Autodesk Inventor part; units mm, degrees
ref_plane "YZ Plane" through (0, 0, 0) normal (1, 0, 0) x (0, 1, 0)
ref_plane "XZ Plane" through (0, 0, 0) normal (0, 1, 0) x (-1, 0, 0)
ref_plane "XY Plane" through (0, 0, 0) normal (0, 0, 1) x (1, 0, 0)
sketch "Sketch1" plane through (0, 0, 0) normal (0, 0, 1) x (1, 0, 0)
  line L0 (0, 0) -> (-375, 0)
  line L1 (-375, 0) -> (-375, -600)
  line L2 (-375, -600) -> (0, -600)
  line L3 (0, -600) -> (0, 0)
  line L4 (-405, 30) -> (30, 30)
  line L5 (30, 30) -> (30, -630)
  line L6 (30, -630) -> (-405, -630)
  line L7 (-405, -630) -> (-405, 30)
  line L8 (-405, -630) -> (-375, -630)
  line L9 (-375, -630) -> (-375, -1270)
  line L10 (-375, -1270) -> (-405, -1270)
  line L11 (-405, -1270) -> (-405, -630)
  line L12 (30, -630) -> (0, -630)
  line L13 (0, -630) -> (0, -1270)
  line L14 (0, -1270) -> (30, -1270)
  line L15 (30, -1270) -> (30, -630)
  line L16 (-375, -1270) -> (0, -1270)
  line L17 (0, -1270) -> (0, -1240)
  line L18 (0, -1240) -> (-375, -1240)
  line L19 (-375, -1240) -> (-375, -1270)
  dimension "d0" = 375
  dimension "d1" = 600
  dimension "d2" = 30
  dimension "d3" = 30
  dimension "d4" = 30
  dimension "d5" = 30
  dimension "d38" = 30
  dimension "d39" = 640
  dimension "d40" = 30
  dimension "d41" = 640
  dimension "d42" = 30
extrude "Extrusion1" add sketch "Sketch1" along normal blind 30 contours L4 L5 L6 L7
sketch "Sketch2" plane through (0, 0, 0) normal (0, 0, -1) x (-1, 0, 0)
  line L0 (375, -600) -> (375, 0)
  line L1 (375, -450) -> (0, -450)
  line L2 (0, -450) -> (0, -410)
  line L3 (0, -410) -> (375, -410)
  line L4 (375, -410) -> (375, -450)
  line L5 (0, -600) -> (375, -600)
  line L6 (202.5, -600) -> (202.5, -450)
  line L7 (172.5, -600) -> (172.5, -450)
  point P0 (0, 0)
  dimension "d8" = 375
  dimension "d9" = 40
  dimension "d10" = 150
extrude "Extrusion2" add sketch "Sketch2" against normal blind 30 contours L1 L2 L3 L0 | L5 L7 L1 L6
sketch "Sketch3" plane through (0, 0, 30) normal (0, 0, 1) x (1, 0, 0)
  line L0 (12.5, -490) -> (17.5, -490)
  line L1 (17.5, -490) -> (17.5, -200)
  line L2 (17.5, -200) -> (12.5, -200)
  line L3 (12.5, -200) -> (12.5, -490)
  line L4 (0, -410) -> (-375, -410)
  line L5 (-392.5, -490) -> (-387.5, -490)
  line L6 (-387.5, -490) -> (-387.5, -200)
  line L7 (-387.5, -200) -> (-392.5, -200)
  line L8 (-392.5, -200) -> (-392.5, -490)
  line L9 (0, -600) -> (-172.5, -600)
  point P0 (0, 0)
  dimension "d13" = 5
  dimension "d14" = 290
  dimension "d18" = 405
  dimension "d37" = 110
extrude "Extrusion3" [suppressed]
sketch "Sketch4" plane through (30, -630, 0) normal (1, 0, 0) x (0, 0, -1)
  line L0 (-30, 0) -> (-30, 660)
  line L1 (-30, 660) -> (-657.8518, 828.2324)
  line L2 (-30, 660) -> (620, 660) construction
  line L3 (-657.8518, 828.2324) -> (-665.6164, 799.2546)
  line L4 (-665.6164, 799.2546) -> (-30, 628.9417)
  point P0 (0, 630)
  dimension "d25" = 650
  dimension "d26" = 165
  dimension "d27" = 30
  dimension "d28" = 270
extrude "Extrusion4" [suppressed]
pattern_linear "Rectangular Pattern1" [suppressed]
sketch "Sketch5" plane through (-375, 0, 30) normal (1, 0, 0) x (0, 0, -1)
  line L0 (-635.6164, 169.2546) -> (-627.8518, 198.2324)
  line L1 (0, -1.0583) -> (-635.6164, 169.2546)
  line L2 (-627.8518, 198.2324) -> (-635.6164, 169.2546)
  line L3 (-635.6164, 169.2546) -> (-606.6386, 161.49)
  line L4 (-606.6386, 161.49) -> (-598.874, 190.4678)
  line L5 (-627.8518, 198.2324) -> (0, 30)
  line L6 (-627.8518, 198.2324) -> (-598.874, 190.4678)
  point P0 (30, 0)
  dimension "d34" = 30
extrude "Extrusion5" [suppressed]
sketch "Sketch6" plane through (0, 0, 0) normal (0, 0, -1) x (-1, 0, 0)
  line L0 (0, -630) -> (0, -1270)
  line L1 (0, -1270) -> (-30, -1270)
  line L2 (-30, -1270) -> (-30, -630)
  line L3 (375, -630) -> (375, -1270)
  line L4 (375, -1270) -> (405, -1270)
  line L5 (405, -1270) -> (405, -630)
  line L6 (0, -1270) -> (375, -1270)
  line L7 (375, -1270) -> (375, -1240)
  line L8 (375, -1240) -> (0, -1240)
  line L9 (0, -1240) -> (0, -1270)
  line L10 (405, 30) -> (405, -630)
  line L11 (-30, -630) -> (-30, 30)
  line L12 (405, -630) -> (375, -630)
  line L13 (405, -630) -> (-30, -630)
  line L14 (0, -630) -> (-30, -630)
  point P0 (0, 0)
  point P1 (405, -1.0583)
  point P2 (-30, -1.0583)
  dimension "d43" = 30
  dimension "d44" = 640
  dimension "d45" = 30
  dimension "d46" = 640
  dimension "d47" = 30
  dimension "d48" = 0
  dimension "d49" = 0
extrude "Extrusion6" add sketch "Sketch6" against normal blind 30 contours L0 L1 L2 L13 | L8 L3 L6 L0 | L12 L5 L4 L3
sketch "Sketch7" plane through (0, 0, 0) normal (0, 0, -1) x (-1, 0, 0)
  circle A0 centre (187.5, -430) radius 40
  point P0 (0, 0)
  dimension "d52" = 80
sketch "Sketch8" plane through (30, -1270, 0) normal (1, 0, 0) x (0, 0, -1)
  line L0 (0, 0) -> (-30, 0)
  line L1 (-30, 0) -> (-311.9078, 102.606)
  line L2 (-30, 0) -> (270, 0) construction
  line L3 (-311.9078, 102.606) -> (-301.6472, 130.7968)
  line L4 (-301.6472, 130.7968) -> (-30, 31.9253)
  line L5 (-30, 640) -> (-30, 30)
  line L6 (-30, 31.9253) -> (-30, 0)
  point P0 (0, 1270)
  dimension "d55" = 300
  dimension "d56" = 160
  dimension "d57" = 30
  dimension "d58" = 90
sketch "Sketch9" plane through (0, -1240, 0) normal (-1, 0, 0) x (0, 0, 1)
  line L0 (311.9078, 72.606) -> (301.6472, 100.7968)
  line L1 (311.9078, 72.606) -> (301.6472, 100.7968)
  line L2 (301.6472, 100.7968) -> (273.4564, 90.5362)
  line L3 (30, 1.9253) -> (301.6472, 100.7968)
  line L4 (273.4564, 90.5362) -> (283.717, 62.3454)
  line L5 (30, -30) -> (311.9078, 72.606)
  line L6 (283.717, 62.3454) -> (311.9078, 72.606)
  point P0 (0, 1240)
  dimension "d64" = 30
sketch "Sketch10" plane through (0, 0, 30) normal (0, 0, 1) x (1, 0, 0)
  line L0 (-405, -1238.0747) -> (-375, -1238.0747)
  line L1 (-405, -1238.0747) -> (30, -1238.0747)
  line L2 (30, -1238.0747) -> (30, -598.0747)
  line L3 (30, -598.0747) -> (-405, -598.0747)
  line L4 (-405, -598.0747) -> (-405, -1238.0747)
  point P0 (0, 0)
  dimension "d67" = 435
  dimension "d68" = 640
sketch "Sketch11" plane through (0, 0, 32) normal (0, 0, 1) x (1, 0, 0)
  line L0 (30, -648.0747) -> (0, -648.0747)
  line L1 (0, -648.0747) -> (0, -678.0747)
  line L2 (0, -678.0747) -> (30, -678.0747)
  line L3 (30, -678.0747) -> (30, -648.0747)
  line L4 (30, -598.0747) -> (-405, -598.0747)
  point P0 (0, 0)
  dimension "d71" = 30
  dimension "d72" = 30
  dimension "d73" = 50
sketch "Sketch12" plane through (0, 0, 382) normal (0, 0, 1) x (1, 0, 0)
  line L0 (-405, -868.0747) -> (-405, -898.0747)
  line L1 (-405, -898.0747) -> (-375, -898.0747)
  line L2 (-375, -898.0747) -> (-375, -868.0747)
  line L3 (-375, -868.0747) -> (-405, -868.0747)
  line L4 (-405, -648.0747) -> (-405, -678.0747)
  line L5 (-405, -678.0747) -> (-375, -678.0747)
  line L6 (-375, -678.0747) -> (-375, -648.0747)
  line L7 (-375, -648.0747) -> (-405, -648.0747)
  line L8 (0, -648.0747) -> (0, -678.0747)
  line L9 (0, -678.0747) -> (30, -678.0747)
  line L10 (30, -678.0747) -> (30, -648.0747)
  line L11 (30, -648.0747) -> (0, -648.0747)
  line L12 (0, -868.0747) -> (0, -898.0747)
  line L13 (0, -898.0747) -> (30, -898.0747)
  line L14 (30, -898.0747) -> (30, -868.0747)
  line L15 (30, -868.0747) -> (0, -868.0747)
  line L16 (-405, -898.0747) -> (-375, -898.0747)
  line L17 (-405, -898.0747) -> (30, -898.0747)
  line L18 (30, -898.0747) -> (30, -648.0747)
  line L19 (30, -648.0747) -> (-405, -648.0747)
  line L20 (-405, -648.0747) -> (-405, -898.0747)
  point P0 (0, 0)
  point P1 (0, -898.0747)
  point P2 (30, -868.0747)
  point P3 (30, -678.0747)
  point P4 (0, -648.0747)
sketch "Sketch13" plane through (-405, -1270, 0) normal (-1, 0, 0) x (0, 0, 1)
  line L0 (232, 591.9253) -> (202, 591.9253)
  line L1 (202, 591.9253) -> (202, 741.9253)
  line L2 (202, 741.9253) -> (232, 741.9253)
  line L3 (232, 741.9253) -> (232, 591.9253)
  line L4 (32, 591.9253) -> (379, 591.9253)
  line L5 (382, 621.9253) -> (382, 371.9253)
  point P0 (0, 1270)
  dimension "d84" = 30
  dimension "d85" = 150
  dimension "d86" = 0
  dimension "d87" = 150
sketch "Sketch14" plane through (-435, -1270, 0) normal (-1, 0, 0) x (0, 0, 1)
  line L0 (232, 741.9253) -> (202, 741.9253)
  line L1 (232, 741.9253) -> (202, 741.9253)
  line L2 (202, 741.9253) -> (202, 711.9253)
  line L3 (202, 711.9253) -> (232, 711.9253)
  line L4 (232, 711.9253) -> (232, 741.9253)
  point P0 (0, 1270)
  point P1 (202, 741.9253)
  dimension "d90" = 30
  dimension "d91" = 30
sketch "Sketch15" plane through (30, -1270, 0) normal (1, 0, 0) x (0, 0, -1)
  line L0 (-657.8518, 1468.2324) -> (-665.6164, 1439.2546) construction
  circle A0 centre (-661.7341, 1453.7435) radius 7.5 construction
  circle A1 centre (-654.5905, 1451.4588) radius 4
  point P0 (0, 1270)
  dimension "d96" = 15
  dimension "d97" = 8
properties part number "rama pod fotel v2 bez mocowań kierownicy"
Can you work these out from the model? Positions are in its coordinate system, mm. A direction names the side the tool comes from. Coordinates: 2 decimals unless noted, no trailing zeros. Order: outer loops, then holes, each group sorted by start corner. A loop starts at its lowest first (then second) coordinate and runs counter-clockwise, first axis right, second up.
1. If we section it at A-A (x = -77): Please give me the cut outline in (y, z), then the cut area to 3 significant figures.
2. For faces 5 (the face through (0, -526, 15)), 6 (the face through (-189, -617, 30)), which set-ups out of +Z, -Z, +X, -X, +Y, -Y let a thin tool reach every point of the face, with its end or its side?
3. If we section it at B-B (y = -1051): Please give me the cut outline in (x, z).
4. I need wall thicknesses on line 1 (Y direction, x = -225, z = 11); line 2 (X direction, y = -521.5, z = 19.5); line 3 (Y direction, x = -184.5, z = 10.75). Which ranges of each line are inside material? Lowest first, please.
5. Thinking about a two-plate mould opening in X: for faces 1 (the face through (-405, -629, 15)), 2 (the face through (-290, -600, 15)), 3 (the face through (-191, -1270, 15)), 4 (the face through (-185, -630, 15)), which applies, +X half, -X half, draft (parallel to the pull), parting line (faces both ways), or undercut?
6. If we section it at C-C (z = 5): Please give me the cut outline in (x, y).
Entries:
1. outline: (-1270, 0) - (-1240, 0) - (-1240, 30) - (-1270, 30) - close; (-630, 0) - (-600, 0) - (-600, 30) - (-630, 30) - close; (-450, 0) - (-410, 0) - (-410, 30) - (-450, 30) - close; (0, 0) - (30, 0) - (30, 30) - (0, 30) - close
1. area: 3,900 mm2
2. face 5: +Z, -Z
2. face 6: +Z, +X, -X, +Y, -Y
3. outline: (-405, 0) - (-375, 0) - (-375, 30) - (-405, 30) - close; (0, 0) - (30, 0) - (30, 30) - (0, 30) - close
4. line 1: y = -1270 to -1240, -630 to -600, -450 to -410, 0 to 30
4. line 2: x = -405 to -375, -202.5 to -172.5, 0 to 30
4. line 3: y = -1270 to -1240, -630 to -410, 0 to 30
5. face 1: -X half
5. face 2: undercut
5. face 3: draft
5. face 4: undercut
6. outline: (-405, -1270) - (30, -1270) - (30, 30) - (-405, 30) - close; hole (-375, -1240) - (0, -1240) - (0, -630) - (-375, -630) - close; hole (-375, -600) - (-202.5, -600) - (-202.5, -450) - (-375, -450) - close; hole (-375, -410) - (0, -410) - (0, 0) - (-375, 0) - close; hole (-172.5, -600) - (0, -600) - (0, -450) - (-172.5, -450) - close
